Could you check a few things on this model? Use its own coordinates, in mm. A direction names the side the tool comes from. Give positions to 0.01 mm unless a question says otherwise; leave off trailing zeros. Write each loop counter-clockwise with the first axis right and the second up, starting at its lowest first coordinate (ties: lowest second). Pieces come first, ordered by that corner, then holes. Notation, with made-up numbers: (-32.75, 70.25) - (3.25, 70.25) arc R17 ccw to (3.25, 97.25) - close; hole circle Ø5 at (54, 71.25). An arc over 180 degrees is marked (long way). Write item = value, one per line.
from build123d import *

# Parameters (mm, degrees)
BOSS_EXTRUDE1_DEPTH  = 20
M4_CLEARANCE_HOLE1_D = 4.5
M4_CLEARANCE_HOLE2_D = 4.5


with BuildPart() as part:
    # Sketch1 → Boss-Extrude1 (new body, symmetric)
    with BuildSketch(Plane(origin=(0, 0, 0), x_dir=(0, 0, -1), z_dir=(1, 0, 0))):
        Polygon((0, 0), (0, 19.05), (1.6, 19.05), (1.6, 1.6), (19.05, 1.6), (19.05, 0), align=None)
    extrude(amount=BOSS_EXTRUDE1_DEPTH, both=True)

    # M4 Clearance Hole1 (through all)
    with Locations(Plane.XY):
        with Locations((-15, 12), (15, 12)):
            Hole(M4_CLEARANCE_HOLE1_D / 2)

    # M4 Clearance Hole2 (through all)
    with Locations(Plane(origin=(0, 0, 0), x_dir=(-1, 0, 0), z_dir=(0, -1, 0))):
        with Locations((-15, 10), (15, 10)):
            Hole(M4_CLEARANCE_HOLE2_D / 2)


solid = part.part
1. If we section it at A-A, the plane x = 15: Please give me the cut outline in (y, z).
Filled sheet:
outline = (0, -19.05) - (1.6, -19.05) - (1.6, -12.25) - (0, -12.25) - close; (0, -7.75) - (1.6, -7.75) - (1.6, -1.6) - (9.75, -1.6) - (9.75, 0) - (0, 0) - close; (14.25, -1.6) - (19.05, -1.6) - (19.05, 0) - (14.25, 0) - close
2. Thinking about a two-plate mould opening in X: for faces 1 (the face through (-20, 1, -5)), 2 (the face through (13.79, 13.897, -0.811)), 3 (the face through (0, 19.05, -1)), which applies, pulls with the +X half, pulls with the -X half, needs draft (parallel to the pull), parting line crosses it, or undercut?
Filled sheet:
face_1 = pulls with the -X half
face_2 = undercut
face_3 = needs draft
3. I need wall thicknesses on line 1 (X direction, y = 1.25, z = -10); line 2 (Z direction, x = -15, y = 1.1); line 3 (Y direction, x = 15, z = -0.4). Which ranges of each line are inside material? Lowest first, please.
Filled sheet:
line_1 = -20 to -17.25, -12.75 to 12.75, 17.25 to 20
line_2 = -19.05 to -12.25, -7.75 to 0
line_3 = 0 to 9.75, 14.25 to 19.05
4. For pin 1 (2 mm diameter, centred on x = 3.5, z = -13.5, fed in from +Y); pin 2 (5 mm diameter, centred on x = 5, y = 9, fed in from -Z), each with a flat end and sliding along its axis, tell me the tip position at first contact or that it passes through.
Filled sheet:
pin_1 = 1.6
pin_2 = -1.6
5. If we section it at B-B, the plane y = 12: Please give me the cut outline in (x, z), and give its area (3 significant figures).
Filled sheet:
outline = (-20, -1.6) - (-17.25, -1.6) - (-17.25, 0) - (-20, 0) - close; (-12.75, -1.6) - (12.75, -1.6) - (12.75, 0) - (-12.75, 0) - close; (17.25, -1.6) - (20, -1.6) - (20, 0) - (17.25, 0) - close
area = 49.6 mm2
6. If we section it at D-D, the plane x = 8: Please give me the cut outline in (y, z), and give its area (3 significant figures).
Filled sheet:
outline = (0, -19.05) - (1.6, -19.05) - (1.6, -1.6) - (19.05, -1.6) - (19.05, 0) - (0, 0) - close
area = 58.4 mm2
7. Which directions (+Z, -Z, +X, -X, +Y, -Y) give clear straight access to the entire face, cutting with the end or side of a thin tool? Please do faces 4 (the face through (0, 10, -1.6)), 5 (the face through (-13.79, 0.811, -11.897)).
Filled sheet:
face_4 = -Z, +X, -X, +Y
face_5 = +Y, -Y
8. If we section it at C-C, the plane z = -10: Please give me the cut outline in (x, y).
Filled sheet:
outline = (-20, 0) - (-17.25, 0) - (-17.25, 1.6) - (-20, 1.6) - close; (-12.75, 0) - (12.75, 0) - (12.75, 1.6) - (-12.75, 1.6) - close; (17.25, 0) - (20, 0) - (20, 1.6) - (17.25, 1.6) - close
